```python
from build123d import *

# Parameters (mm, degrees)
SKETCH1_R           = 11.500000000000005
SKETCH1_R_2         = 5
BOSS_EXTRUDE1_DEPTH = 3
FILLET1_R           = 1


with BuildPart() as part:
    # Sketch1 → Boss-Extrude1 (new body)
    # profile 1 of 2: a face of its own
    with BuildSketch(Plane(origin=(0, 0, 0), x_dir=(1, 0, 0), z_dir=(0, 1, 0))):
        with BuildLine():
            ThreePointArc((11.500000000000005, 40), (-2.11e-15, 28.499999999999993), (-11.500000000000005, 40))
            Line((-11.500000000000002, 40), (-11.5, 0))
            ThreePointArc((-11.5, 1.41e-15), (7e-16, 11.5), (11.5, 0))
            Line((11.5, 0), (11.500000000000002, 40))
        make_face()
    # profile 2 of 2: a face of its own
    with BuildSketch(Plane(origin=(0, 0, 0), x_dir=(1, 0, 0), z_dir=(0, 1, 0))):
        with Locations((0, 40)):
            Circle(SKETCH1_R)
        with Locations(Location((0, 40, 0), (0, 0, 270))):
            Circle(SKETCH1_R_2, mode=Mode.SUBTRACT)
    extrude(amount=BOSS_EXTRUDE1_DEPTH)

    # Fillet1
    fillet1_edges = [part.edges().sort_by_distance(p)[0] for p in [
        (11.5, 1.5, -1.22e-15),
        (-11.5, 1.5, -7e-16),
    ]]
    fillet(fillet1_edges, radius=FILLET1_R)


solid = part.part
```
Work out the finished part from the listing and answer in its coordinate system (mm). Coordinates: 2 decimals unless noted, no trailing zeros. Loops run counter-clockwise (first coordinate to the right, second up) from the corner with the lowest first, then second, coordinate; pieces in that order, holes last.
1) Section C-C (z = -10.5) is taken. Give the vertices of the cut face in (x, y), plus the area to 3 significant figures.
Results:
outline: (-11.5, 0) - (-4.69, 0) - (-4.69, 3) - (-11.5, 3) - close; (4.69, 0) - (11.5, 0) - (11.5, 3) - (4.69, 3) - close
area: 40.9 mm2
2) For a pull along X with two mould halves and no side action, classify faces 1 (the flat face through (-11.5, 1, -24)), 2 (the cylindrical face through (-10.8, 1.52, -5.83)), 3 (the flat face through (0, 3, -29)) as +X half, -X half, draft (parallel to the pull), parting line (faces both ways), or undercut.
Results:
face 1: -X half
face 2: undercut
face 3: draft
3) Flat-ended cylindrical pins translate along their axes: pin 1 (9 mm diameter, centred on x = 0, z = -40, fed in from +Y); pin 2 (1.5 mm diameter, centred on x = -2, y = 2, fed in from +Z). Find the tip coordinate at first contact, or state that the pin passes through.
Results:
pin 1: passes through
pin 2: stops at z = -11.17
4) Consider probe 1 along X at (y, z) = (1.75, -40); probe 2 along Z at (x, y) = (1.75, 1.9); probe 3 along X at (y, z) = (2.8, -36). Determine where each line is inside the solid, lowest interval first.
Results:
probe 1: x = -11.5 to -5, 5 to 11.5
probe 2: z = -51.37 to -44.68, -35.32 to -11.37
probe 3: x = -11.5 to -3, 3 to 11.5
5) Section D-D (x = 10.25) is taken. Give the vertices of the cut face in (y, z), plus the area to 3 significant figures.
Results:
outline: (0, -45.21) - (3, -45.21) - (3, -5.81) - (0, -5.81) - close
area: 118 mm2
6) Section B-B (y = 0.9) is taken. Give the vertices of the cut face in (x, z).
Results:
outline: (-11.5, -40) arc R11.5 ccw to (11.5, -40) - (11.5, -6.78) arc R1 ccw to (9.66, -6.24) arc R11.5 cw to (-9.66, -6.24) arc R1 ccw to (-11.5, -6.78) - close; hole circle Ø10 at (0, -40)
7) Section A-A (x = 0) is taken. Give the vertices of the cut face in (y, z).
Results:
outline: (0, -51.5) - (3, -51.5) - (3, -45) - (0, -45) - close; (0, -35) - (3, -35) - (3, -11.5) - (0, -11.5) - close
